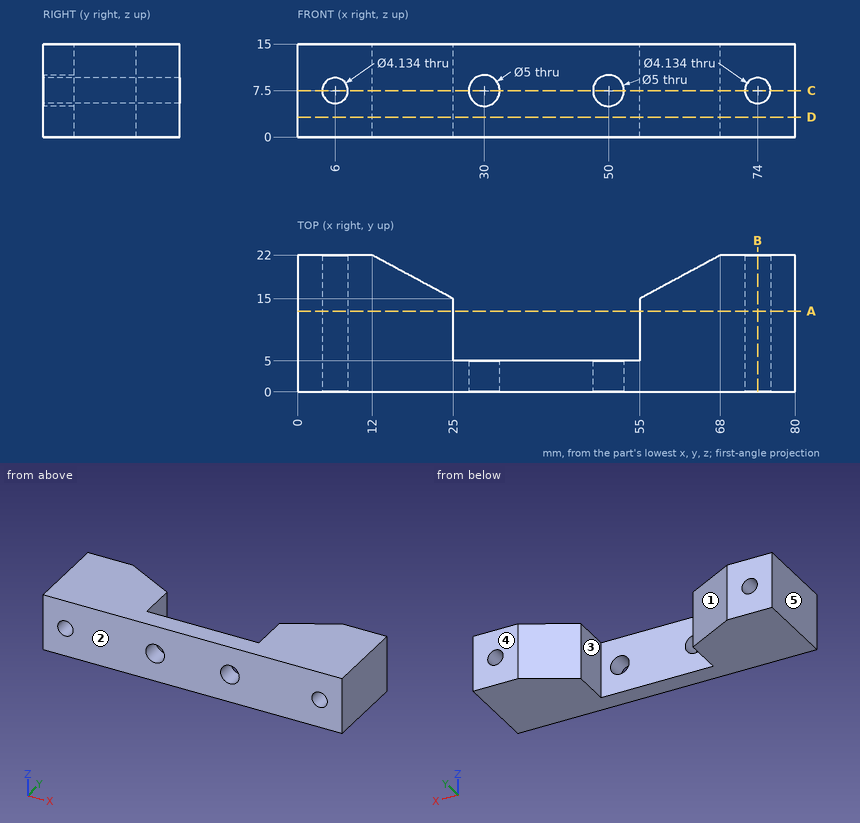
Design review of the part shown in the three views and the two pictorial views. Dimensions are in mm from the part's minimum x, y and z. A direction names the side the tool comes from. Round coordinates to 2 decimals unless told otherwise and drop trailing zeros. Write each loop counter-clockwise with the first axis right and the second up, starting at its lowest first coordinate (ties: lowest second). Pieces come first, ordered by that corner, then holes.
Item 1: Consider section C-C on z = 7.5. Give the boundary of the cut face in (x, y), and give its area (3 significant figures).
Item 2: For pin 1 Ø4.5 at (x, z) = (47, 8.5) entering from +Y, flat-tipped, find the tip position at first contact; note if it passes through.
Item 3: For the marked faces 1 and 2, list the 3-axis set-ups (+Z, -Z, +X, -X, +Y, -Y) from which the entire face can be reached by the end or side of a thin tool; tool diameter is ignored.
Item 4: Consider section D-D on z = 3.25. Give the boundary of the cut face in (x, y).
Item 5: Wall thickness on L1, parallel to X at y = 9.5, z = 10; L2, parallel to Z at x = 6, y = 10.25; L3, parallel to Z at x = 50, y = 2.8: over which ranges is each line inside the solid? List them lowest first.
Item 6: Draft analysis for pull direction X (two halves, no side actions). For the marked faces 3, 4 and 5, state which applies: released by +X, released by -X, zero draft, split by the parting line, or undercut.
Item 7: Consider section B-B on x = 74. Give the boundary of the cut face in (y, z).
Item 8: Consider section A-A on y = 13. Give the boundary of the cut face in (x, z), and give its area (3 significant figures).
Check values:
1. outline: (0, 0) - (3.93, 0) - (3.93, 22) - (0, 22) - close; (8.07, 0) - (27.5, 0) - (27.5, 5) - (25, 5) - (25, 15) - (12, 22) - (8.07, 22) - close; (32.5, 0) - (47.5, 0) - (47.5, 5) - (32.5, 5) - close; (52.5, 0) - (71.93, 0) - (71.93, 22) - (68, 22) - (55, 15) - (55, 5) - (52.5, 5) - close; (76.07, 0) - (80, 0) - (80, 22) - (76.07, 22) - close
1. area: 927 mm2
2. pin 1: stops at y = 5
3. face 1: +Z, -Z, +Y
3. face 2: +Z, -Z, +X, -X, -Y
4. outline: (0, 0) - (80, 0) - (80, 22) - (68, 22) - (55, 15) - (55, 5) - (25, 5) - (25, 15) - (12, 22) - (0, 22) - close
5. L1: x = 0 to 25, 55 to 80
5. L2: z = 0 to 5.43, 9.57 to 15
5. L3: z = 0 to 5, 10 to 15
6. face 3: undercut
6. face 4: zero draft
6. face 5: released by -X
7. outline: (0, 0) - (22, 0) - (22, 5.43) - (0, 5.43) - close; (0, 9.57) - (22, 9.57) - (22, 15) - (0, 15) - close
8. outline: (0, 0) - (25, 0) - (25, 15) - (0, 15) - close; (55, 0) - (80, 0) - (80, 15) - (55, 15) - close; hole circle Ø4.13 at (6, 7.5); hole circle Ø4.13 at (74, 7.5)
8. area: 723 mm2
